from build123d import *

# Parameters (mm, degrees)
PAD_DEPTH    = 20
POCKET_DEPTH = 258.663147
FILLET_R     = 4


with BuildPart() as part:
    # Sketch → Pad (new body, symmetric)
    with BuildSketch(Plane.XZ):
        with BuildLine():
            Line((0, 23), (0, 0))
            Line((0, 0), (65, 0))
            Line((65, 0), (65, 12.5))
            ThreePointArc((65, 12.5), (64.267767, 14.267767), (62.5, 15))
            Line((47.5, 15), (62.5, 15))
            Line((32.5, 15), (47.5, 15))
            Line((32.5, 15), (28.584863, 37.889336))
            ThreePointArc((28.584863, 37.889336), (18.697717, 55.167439), (0, 62))
            Line((0, 43), (0, 62))
            ThreePointArc((0, 23), (10, 33), (0, 43))
        make_face()
    pad = extrude(amount=PAD_DEPTH, both=True)

    # Sketch001 → Pocket (cut, through all)
    with BuildSketch(Plane.XY):
        with BuildLine():
            ThreePointArc((45, 5), (40, 0), (45, -5))
            Line((45, -5), (50, -5))
            ThreePointArc((50, -5), (55, 0), (50, 5))
            Line((50, 5), (45, 5))
        make_face()
    pocket = extrude(amount=POCKET_DEPTH, mode=Mode.SUBTRACT)

    # Mirrored: Pad, Pocket across Sketch V_Axis
    add(pad.mirror(Plane(origin=(0, 0, 0), x_dir=(0, -1, 0), z_dir=(1, 0, 0))))
    add(pocket.mirror(Plane(origin=(0, 0, 0), x_dir=(0, -1, 0), z_dir=(1, 0, 0))), mode=Mode.SUBTRACT)

    # Fillet
    fillet_edges = [part.edges().sort_by_distance(p)[0] for p in [
        (65, -20, 6.25),
        (65, 20, 6.25),
    ]]
    fillet(fillet_edges, radius=FILLET_R)


solid = part.part
Could you check a few things on this model? Use its own coordinates, in mm. A direction names the side the tool comes from. Give positions to 0.01 mm unless a question says otherwise; leave off trailing zeros. Order: outer loops, then holes, each group sorted by start corner. A loop starts at its lowest first (then second) coordinate and runs counter-clockwise, first axis right, second up. Notation, with made-up numbers: (9.25, -29) -> (56.25, -29) arc R10 ccw to (56.25, -19) -> close; hole circle Ø2 at (63.5, 3). An arc over 180 degrees is marked (long way). Answer in a Markdown table with one row per item. Add a question column.
Item 1: Imagine slicing it at D-D (z = 8). List the corners of the cut face in (x, y) for me.
Item 2: Imagine slicing it at A-A (x = 3). List the corners of the cut face in (y, z) for me, and give its area (3 significant figures).
Item 3: Imagine slicing it at B-B (z = 33). List the corners of the cut face in (x, y) for me.
Item 4: We'd pull the mould along Y, two halves only. Please class faces 4 (the cylindrical face through (-40, 0, 7)), 5 (the cylindrical face through (64.287, -0.224, 14.248)), 6 (the cylindrical face through (47.29, -18.859, 13.797)), 7 (the flat face through (47, -5, 7)): pulls with the +Y half, pulls with the -Y half, needs draft (parallel to the pull), parting line crosses it, or undercut.
Item 5: For faces 1 (the cylindrical face through (47.29, 18.859, 13.797)), 2 (the flat face through (48, 5, 7)), 3 (the flat face through (-54, -5, 15)), which set-ups out of +Z, -Z, +X, -X, +Y, -Y let a thin tool reach every point of the face, with its end or its side?
Item 6: I'm going to push flat-ended pins straight in: P1, Ø12, axis at y = 7.5, z = 49, coming from the -X side; P2, Ø18, axis at x = 0, z = 33, coming from the +Y side; P3, Ø10, axis at y = 0.5, z = 41, coming from the -X side; P4, Ø3, axis at y = 5.5, z = 50, coming from the -X side. Where does each tip first touch, or does it pass through?
Item 7: Please list where these lines run through material, in increasing order: probe 1 along X at (y, z) = (3, 8); probe 2 along X at (y, z) = (1.5, 3.5); probe 3 along Z at (x, y) = (57.5, 15).
Item 8: Imagine slicing it at C-C (y = 13). List the corners of the cut face in (x, z) for me.
Result:
| question | item | result |
|---|---|---|
| 1 | outline | (-65, -20) -> (61, -20) arc R4 ccw to (65, -16) -> (65, 16) arc R4 ccw to (61, 20) -> (-65, 20) -> close; hole (-50, -5) -> (-45, -5) arc R5 ccw to (-45, 5) -> (-50, 5) arc R5 ccw to start; hole (45, -5) -> (50, -5) arc R5 ccw to (50, 5) -> (45, 5) arc R5 ccw to start |
| 2 | outline | (-20, 0) -> (20, 0) -> (20, 23.46) -> (-20, 23.46) -> close; (-20, 42.54) -> (20, 42.54) -> (20, 61.84) -> (-20, 61.84) -> close |
| 2 | area | 1,710 mm2 |
| 3 | outline | (-29.42, -20) -> (-10, -20) -> (-10, 20) -> (-29.42, 20) -> close; (10, -20) -> (29.42, -20) -> (29.42, 20) -> (10, 20) -> close |
| 4 | face 4 | undercut |
| 4 | face 5 | needs draft |
| 4 | face 6 | pulls with the -Y half |
| 4 | face 7 | undercut |
| 5 | face 1 | +Z, +X, +Y |
| 5 | face 2 | +Z, -Z |
| 5 | face 3 | +Z, -X, +Y, -Y |
| 6 | P1 | x = -27.22 |
| 6 | P2 | through |
| 6 | P3 | x = -28.91 |
| 6 | P4 | x = -24.51 |
| 7 | probe 1 | -65 to -54, -41 to 41, 54 to 65 |
| 7 | probe 2 | -65 to -54.77, -40.23 to 40.23, 54.77 to 65 |
| 7 | probe 3 | 0 to 15 |
| 8 | outline | (-65, 0) -> (65, 0) -> (65, 12.5) arc R2.5 ccw to (62.5, 15) -> (32.5, 15) -> (28.58, 37.89) arc R29 ccw to (0, 62) arc R29 ccw to (-28.58, 37.89) -> (-32.5, 15) -> (-62.5, 15) arc R2.5 ccw to (-65, 12.5) -> close; hole circle Ø20 at (0, 33) |
